Could you check a few things on this model? Use its own coordinates, in mm. Face numbers are marked on the shaded views. A direction names the side the tool comes from. Coordinates: 2 decimals unless noted, no trailing zeros. Order: outer loops, then holes, each group sorted by start corner. A loop starts at its lowest first (then second) coordinate and runs counter-clockwise, first axis right, second up. Notation, with made-up numbers: (-6.5, 62.5) - (3.5, 62.5) arc R18 cw to (3.5, 97.5) - close; hole circle Ø7 at (14, 36.5). An arc over 180 degrees is marked (long way). One line per item, written item: value.
from build123d import *

# Parameters (mm, degrees)
SKETCH2_R             = 85
BOSS_EXTRUDE1_DEPTH   = 50
SKETCH3_R             = 60
BOSS_EXTRUDE2_DEPTH   = 5
BOSS_EXTRUDE3_START   = 5
SKETCH4_R             = 60
BOSS_EXTRUDE3_DEPTH   = 5
SKETCH5_R             = 5
CUT_EXTRUDE1_DEPTH    = 100
BODY_MOVE_COPY1_ANGLE = 90
FILLET1_R             = 5
FILLET2_R             = 12


with BuildPart() as part:
    # Sketch2 → Boss-Extrude1 (new body)
    with BuildSketch(Plane(origin=(0, 0, 0), x_dir=(1, 0, 0), z_dir=(0, 1, 0))):
        with Locations(Location((0, 0, 0), (0, 0, 270))):
            Circle(SKETCH2_R)
    extrude(amount=BOSS_EXTRUDE1_DEPTH)

    # Sketch3 → Boss-Extrude2 (add)
    with BuildSketch(Plane(origin=(0, 50, 0), x_dir=(1, 0, 0), z_dir=(0, 1, 0))):
        with Locations(Location((0, 0, 0), (0, 0, 270))):
            Circle(SKETCH3_R)
    extrude(amount=BOSS_EXTRUDE2_DEPTH)

    # Sketch4 → Boss-Extrude3 (add)
    with BuildSketch(Plane.XZ.offset(BOSS_EXTRUDE3_START)):
        with Locations(Location((0, 0, 0), (0, 0, 90))):
            Circle(SKETCH4_R)
    extrude(amount=-BOSS_EXTRUDE3_DEPTH)

    # Sketch5 → Cut-Extrude1 (cut)
    with BuildSketch(Plane(origin=(0, 55, 0), x_dir=(1, 0, 0), z_dir=(0, 1, 0))):
        with Locations(Location((0, 0, 0), (0, 0, 270))):
            Circle(SKETCH5_R)
    extrude(amount=-CUT_EXTRUDE1_DEPTH, mode=Mode.SUBTRACT)


with BuildPart() as part_1:
    # Body-Move/Copy1: moved
    add(part.part.rotate(Axis((0, 10, 0), (1, 0, 0)), BODY_MOVE_COPY1_ANGLE))

    # Fillet1
    fillet1_edges = [part_1.edges().sort_by_distance(p)[0] for p in [
        (0, 70, -15),
        (0, 70, 45),
    ]]
    fillet(fillet1_edges, radius=FILLET1_R - 0.0001)  # a hair under: the kernel refuses the full size

    # Fillet2
    fillet2_edges = [part_1.edges().sort_by_distance(p)[0] for p in [
        (0, 95, -10),
        (0, 95, 40),
        (0, 70, 40),
    ]]
    fillet(fillet2_edges, radius=FILLET2_R)


solid = part_1.part
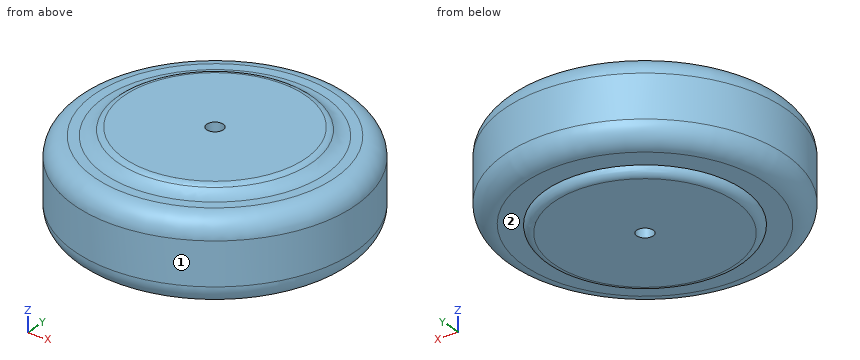
Item 1: For the marked faces 1 and 2, which set-ups out of +Z, -Z, +X, -X, +Y, -Y let a thin tool reach every point of the face, with its end or its side?
Conclusion:
face 1: +Z, -Z
face 2: -Z
Item 2: I want a section at A-A on z = 15.5. Please give me the cut outline in (x, y), then the cut area to 3 significant figures.
Conclusion:
outline: circle Ø170 at (0, 10); hole circle Ø10 at (0, 10)
area: 22,600 mm²
Item 3: I want a section at B-B on z = 35.5. Please give me the cut outline in (x, y) (1 decimal), then the cut area to 3 significant figures.
Conclusion:
outline: circle Ø164.7 at (0, 10); hole circle Ø10 at (0, 10)
area: 21,200 mm²
Item 4: I'm going to push flat-ended pins straight in: pin 1 Ø4 at (y, z) = (64, 7) entering from +X; pin 2 Ø5 at (y, z) = (18.5, 24.5) entering from -X; pin 3 Ø3 at (x, z) = (-36.5, -2.5) entering from +Y. Where does each tip first touch, or does it pass through?
Conclusion:
pin 1: x = 67.24
pin 2: x = -84.79
pin 3: y = 86.72
Item 5: If I drill on probe 1 along X at (y, z) = (10, 16); probe 2 along Z at (x, y) = (-53, -38.5); probe 3 along X at (y, z) = (-40, 33.5), over which ranges is the centre line in solid material (lowest first)?
Conclusion:
probe 1: -85 to -5, 5 to 85
probe 2: -10 to 40
probe 3: -67.08 to 67.08
